Design review of the part shown in the three views and the two pictorial views. Dimensions are in mm from the part's minimum x, y and z. A direction names the side the tool comes from. Give positions to 0.01 mm unless a question says otherwise; leave off trailing zeros. Loops run counter-clockwise (first coordinate to the right, second up) from the corner with the lowest first, then second, coordinate; pieces in that order, holes last. Notation, with made-up numbers: (10.5, -28) -> (61.5, -28) arc R29 ccw to (61.5, -6) -> close; hole circle Ø1 at (-11, -21.75). An arc over 180 degrees is marked (long way). Answer as CSV lines item,"result".
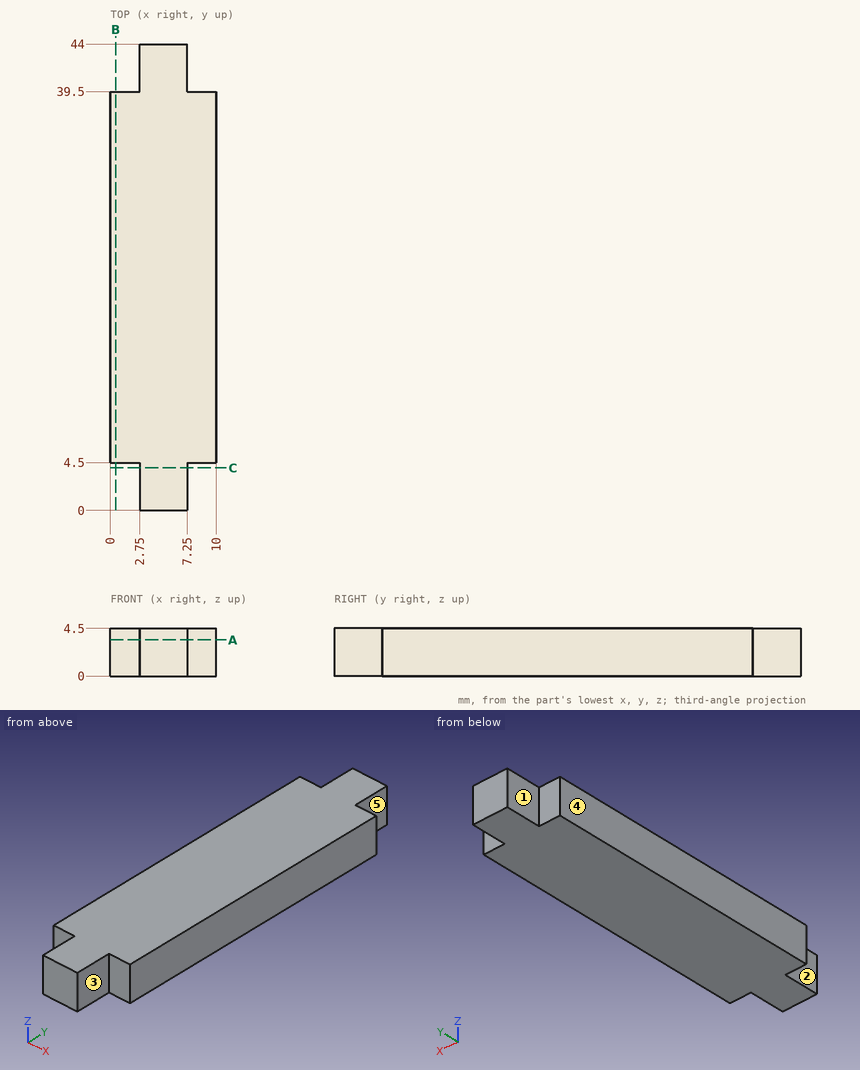
Q1. We need section B-B, the plane x = 0.5. State the section outline as (y, z) points.
Filled sheet:
outline,"(4.5, 0) -> (39.5, 0) -> (39.5, 4.5) -> (4.5, 4.5) -> close"
Q2. Clearance check with flat-ended pins moving along their axes: pin 1 Ø1.4 at (x, z) = (8, 2) entering from +Y; pin 2 Ø2 at (x, z) = (9, 3) entering from -Y; pin 3 Ø1.3 at (y, z) = (42, 1) entering from -X; pin 4 Ø5 at (x, y) = (7, 10) entering from -Z. State where each tip first meets the part, or that it passes through.
Filled sheet:
pin 1,"stops at y = 39.5"
pin 2,"stops at y = 4.5"
pin 3,"stops at x = 2.75"
pin 4,"stops at z = 0"
Q3. We need section A-A, the plane z = 3.4. State the section outline as (x, y) points, and give its area (4 significant figures).
Filled sheet:
outline,"(0, 4.5) -> (2.75, 4.5) -> (2.75, 0) -> (7.25, 0) -> (7.25, 4.5) -> (10, 4.5) -> (10, 39.5) -> (7.25, 39.5) -> (7.25, 44) -> (2.75, 44) -> (2.75, 39.5) -> (0, 39.5) -> close"
area,"390.5 mm^2"
Q4. We need section C-C, the plane y = 4. State the section outline as (x, z) points, and give its area (4 significant figures).
Filled sheet:
outline,"(2.75, 0) -> (7.25, 0) -> (7.25, 4.5) -> (2.75, 4.5) -> close"
area,"20.25 mm^2"
Q5. For the marked faces 1, 2, 3, 4 and 5, list the 3-axis set-ups (+Z, -Z, +X, -X, +Y, -Y) from which the entire face can be reached by the end or side of a thin tool; tool diameter is ignored.
Filled sheet:
face 1,"+Z, -Z, -X, +Y"
face 2,"+Z, -Z, -X, -Y"
face 3,"+Z, -Z, +X, -Y"
face 4,"+Z, -Z, -X, +Y, -Y"
face 5,"+Z, -Z, +X, +Y"
Q6. To check wall thickness, follow probe 1 along Y at (x, z) = (1, 2.8); probe 2 along X at (y, z) = (3.5, 3). State the ranges of each line that lie inside material, in increasing order. Write a range as from..to.
Filled sheet:
probe 1,"y = 4.5..39.5"
probe 2,"x = 2.75..7.25"
